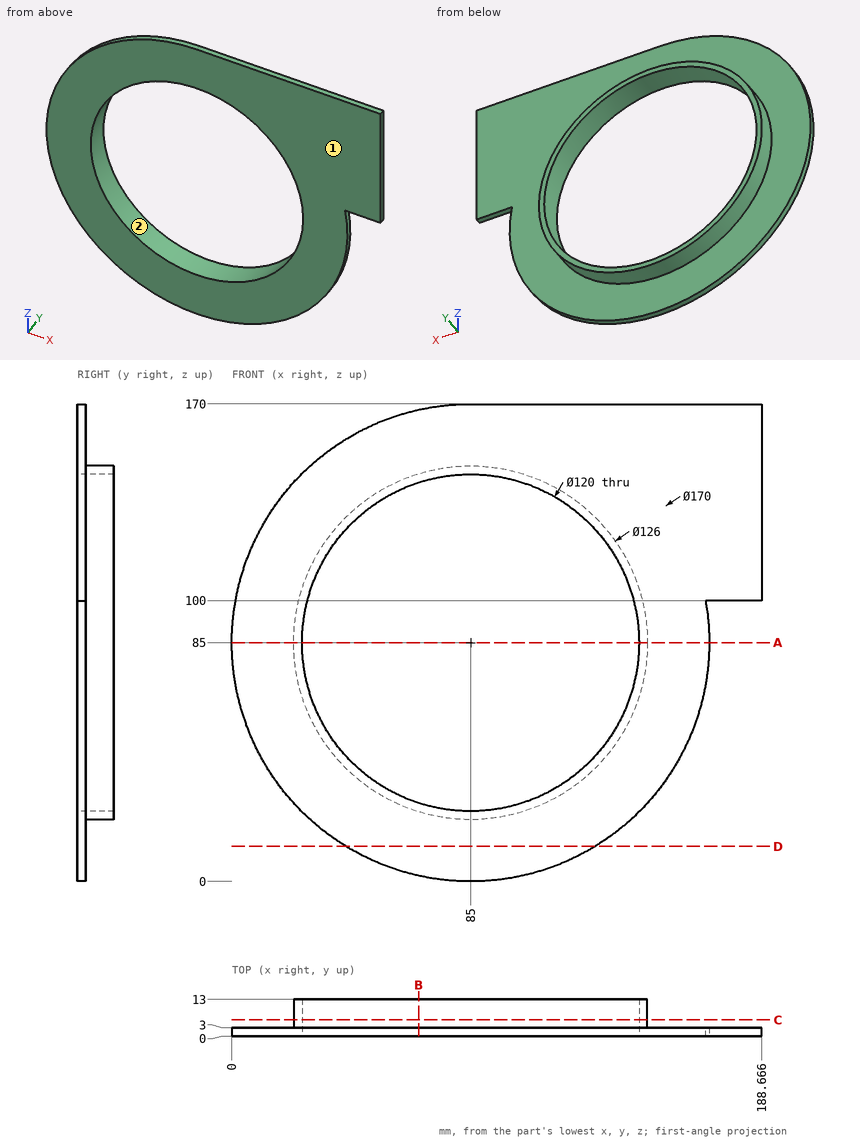
Geometry: see drawing. Coordinates: mm, zero at the bounding-box minimum. Round coordinates to 2 decimals unless told otherwise and drop trailing zeros. Write each loop counter-clockwise with the first axis right and the second up, starting at its lowest first coordinate (ties: lowest second). Pieces come first, ordered by that corner, then holes.
Item 1: Mould query, pull axis X, two halves, no side actions, for the marked faces 1 and 2. Classes: +X half, -X half, draft (parallel to the pull), parting line (faces both ways), or undercut.
Item 2: Material intervals for L1, parallel to X at y = 9.5, z = 85; L2, parallel to Y at x = 47, z = 158.5, sorted ascending.
Item 3: Section query C-C (y = 5.75). Return loops of the section in (x, z), plus the area to 3 significant figures.
Item 4: Section query B-B (x = 66.5). Return loops of the section in (y, z).
Item 5: Section query A-A (z = 85). Return loops of the section in (x, y).
Item 6: Pin query (flat end, axial travel): P1, Ø3, axis at y = 7.5, z = 100, coming from the -X side; P2, Ø6, axis at y = 7, z = 41.5, coming from the +X side; P3, Ø1, axis at y = 10, z = 81, coming from the -X side. Return the tip coordinate at first contact, or that it passes through.
Item 7: Section query D-D (z = 12.5). Return loops of the section in (x, y), plus the area to 3 significant figures.
Completed:
1. face 1: draft
1. face 2: undercut
2. L1: x = 22 to 25, 145 to 148
2. L2: y = 0 to 3
3. outline: circle Ø126 at (85, 85); hole circle Ø120 at (85, 85)
3. area: 1,160 mm2
4. outline: (0, 2.04) - (3, 2.04) - (3, 24.78) - (13, 24.78) - (13, 27.92) - (0, 27.92) - close; (0, 142.08) - (13, 142.08) - (13, 145.22) - (3, 145.22) - (3, 167.96) - (0, 167.96) - close
5. outline: (0, 0) - (25, 0) - (25, 13) - (22, 13) - (22, 3) - (0, 3) - close; (145, 0) - (170, 0) - (170, 3) - (148, 3) - (148, 13) - (145, 13) - close
6. P1: stops at x = 23.46
6. P2: stops at x = 133.26
6. P3: stops at x = 22.1
7. outline: (40.63, 0) - (129.37, 0) - (129.37, 3) - (40.63, 3) - close
7. area: 266 mm2
